Could you check a few things on this model? Use its own coordinates, in mm. A direction names the side the tool comes from. Round coordinates to 2 decimals unless told otherwise and drop trailing zeros. Loops run counter-clockwise (first coordinate to the right, second up) from the corner with the lowest first, then second, coordinate; pieces in that order, holes last. Notation, with made-up numbers: (21, 28) - (27, 28) arc R15 ccw to (27, 40) - close; hole circle Ø6 at (-25, -19). An arc over 180 degrees is marked (long way). Answer as CSV lines item,"result". Start each with the question number.
1) Suppose I cut it at A-A, the plane x = 0. Write out the boundary of the cut face in (y, z).
2) I'm going to push flat-ended pins straight in: pin 1 Ø3 at (y, z) = (2.5, -8) entering from +X; pin 2 Ø3 at (y, z) = (5, 0) entering from +X; pin 3 Ø2 at (x, y) = (-6.5, 12) entering from -Z; pin 4 Ø1.5 at (x, y) = (-17.5, 1.5) entering from -Z. Where does each tip first touch, or does it pass through?
3) Suppose I cut it at B-B, the plane z = 0. Write out the boundary of the cut face in (x, y).
4) Which directions (+Z, -Z, +X, -X, +Y, -Y) give clear straight access to the entire face, cutting with the end or side of a thin tool? Please do faces 1 (the face through (-32.97, 3.78, 0.27)), 2 (the face through (0, 14, 0)).
5) We'd pull the mould along Z, two halves only. Please class faces 3 (the face through (33.71, 7.89, -4.43)), 4 (the face through (-1.551, 14.986, -20.008)), 5 (the face through (0.27, 3.78, 32.97)): pulls with the +Z half, pulls with the -Z half, needs draft (parallel to the pull), parting line crosses it, or undercut.
6) Please list where these lines run through material, in increasing order: line 1 along Y through (x, z) = (0, 33.15); line 2 along Y through (x, z) = (-30, 3); line 3 along Z through (x, y) = (0, 9.5).
7) Suppose I cut it at C-C, the plane y = 5. Count the separate pieces of the cut face and the enclosed holes in it, then the cut area to 3 significant figures.
8) Suppose I cut it at D-D, the plane z = 14. Write out the boundary of the cut face in (x, y).
```python
from build123d import *

# Parameters (mm, degrees)
SKETCH_1_R               = 34
EXTRUDE_1_DEPTH          = 16
CUT_EXTRUDE_1_REACH      = 52.675
CUT_EXTRUDE_1_END_RADIUS = 34
SKETCH_2_R               = 1.25
PATTERN_CIRCULAR_1_COUNT = 8
SKETCH_3_R               = 32
CUT_EXTRUDE_2_DEPTH      = 14
SKETCH_5_R               = 1.748779673
CUT_EXTRUDE_3_DEPTH      = 51.675438003


with BuildPart() as part:
    # 草图1 → 凸台-拉伸1 (new body)
    with BuildSketch(Plane(origin=(0, 0, 0), x_dir=(1, 0, 0), z_dir=(0, 1, 0))):
        with Locations(Location((0, 0, 0), (0, 0, 270))):
            Circle(SKETCH_1_R)
    extrude(amount=EXTRUDE_1_DEPTH)

    # 切除-拉伸1: up to this cylinder (the profile starts inside it)
    cut_extrude_1_end = Plane(origin=(0, 5, 0), z_dir=(0, -1, 0)) * Cylinder(CUT_EXTRUDE_1_END_RADIUS, 174.35, mode=Mode.PRIVATE)
    # 草图2 → 切除-拉伸1 (cut, up to the surface)
    with BuildSketch(Plane.XY, mode=Mode.PRIVATE) as cut_extrude_1_sk1:
        with Locations((0, 5)):
            Circle(SKETCH_2_R)
    cut_extrude_1_tool1 = extrude(cut_extrude_1_sk1.sketch, amount=-CUT_EXTRUDE_1_REACH, mode=Mode.PRIVATE) & cut_extrude_1_end
    cut_extrude_1 = cut_extrude_1_tool1.solids().sort_by_distance((0, 5, 0))[0]
    add(cut_extrude_1, mode=Mode.SUBTRACT)

    # 阵列(圆周)1: 切除-拉伸1 ×8 about axis
    pattern_circular_1_axis = Axis((0, 16, 0), (0, 1, 0))
    for i in range(1, PATTERN_CIRCULAR_1_COUNT):
        add(cut_extrude_1.rotate(pattern_circular_1_axis, i * 360 / PATTERN_CIRCULAR_1_COUNT), mode=Mode.SUBTRACT)

    # 草图3 → 切除-拉伸2 (cut)
    with BuildSketch(Plane(origin=(0, 0, 0), x_dir=(1, 0, 0), z_dir=(0, 1, 0))):
        with Locations(Location((0, 0, 0), (0, 0, 270))):
            Circle(SKETCH_3_R)
    extrude(amount=CUT_EXTRUDE_2_DEPTH, mode=Mode.SUBTRACT)

    # 草图5 → 切除-拉伸3 (cut, through all)
    with BuildSketch(Plane(origin=(0, 0, 0), x_dir=(1, 0, 0), z_dir=(0, 1, 0))):
        with Locations(Location((0, 20.814842856, 0), (0, 0, 270))):
            Circle(SKETCH_5_R)
    extrude(amount=CUT_EXTRUDE_3_DEPTH, mode=Mode.SUBTRACT)


solid = part.part
```
Filled sheet:
1,outline,"(0, -34) - (3.75, -34) - (3.75, -32) - (0, -32) - close; (0, 32) - (3.75, 32) - (3.75, 34) - (0, 34) - close; (6.25, -34) - (16, -34) - (16, -22.56) - (14, -22.56) - (14, -32) - (6.25, -32) - close; (6.25, 32) - (14, 32) - (14, -19.07) - (16, -19.07) - (16, 34) - (6.25, 34) - close"
2,pin 1,"x = 33.37"
2,pin 2,"x = 34"
2,pin 3,"z = -33.55"
2,pin 4,"z = -29.59"
3,outline,"(-34, 0) - (-32, 0) - (-32, 3.75) - (-34, 3.75) - close; (-34, 6.25) - (-32, 6.25) - (-32, 14) - (32, 14) - (32, 6.25) - (34, 6.25) - (34, 16) - (-34, 16) - close; (32, 0) - (34, 0) - (34, 3.75) - (32, 3.75) - close"
4,face 1,"+X, -X"
4,face 2,"-Y"
5,face 3,"parting line crosses it"
5,face 4,"undercut"
5,face 5,"needs draft"
6,line 1,"0 to 3.75, 6.25 to 16"
6,line 2,"14 to 16"
6,line 3,"-34 to -32, 32 to 34"
7,separate pieces,"8"
7,enclosed holes,"0"
7,area,"375 mm²"
8,outline,"(-30.98, 0) - (-28.77, 0) - (-28.77, 14) - (28.77, 14) - (28.77, 0) - (30.98, 0) - (30.98, 16) - (-30.98, 16) - close"
